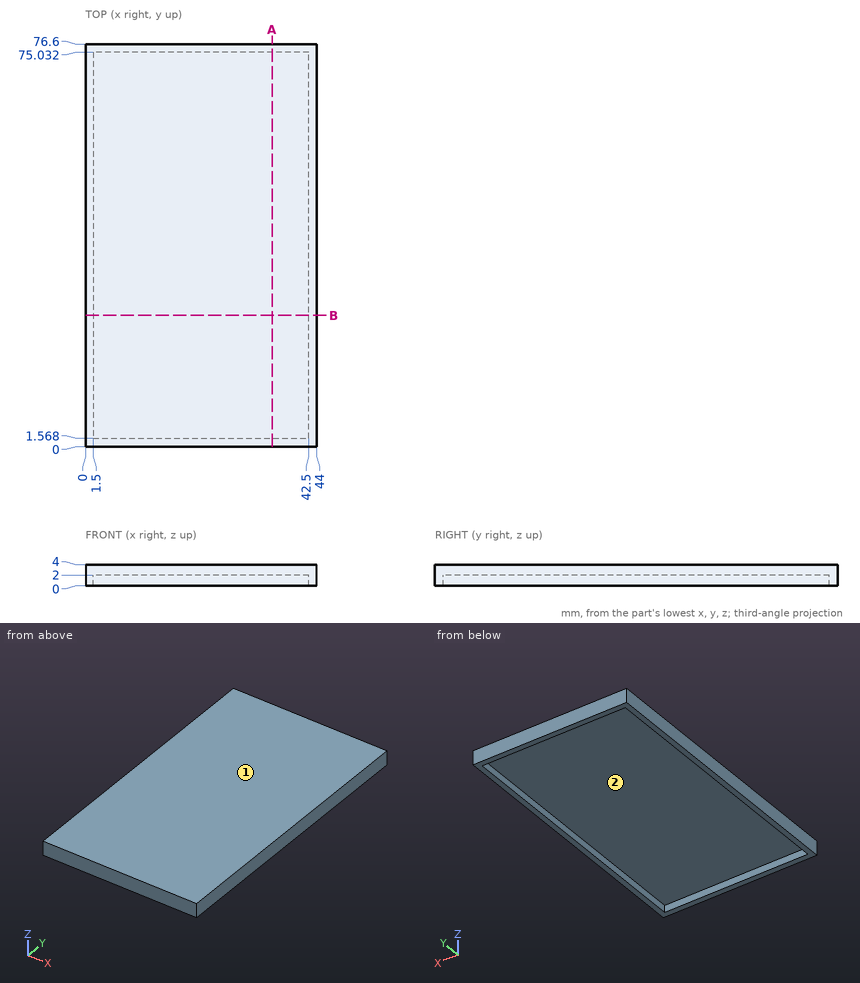
Can you work these out from the drawing? Everything is in mm from the part's minimum corner. Give positions to 0.01 mm unless a question says otherwise; leave off trailing zeros. Order: outer loops, then holes, each group sorted by start corner. A loop starts at its lowest first (then second) coordinate and runs counter-clockwise, first axis right, second up. Notation, with made-up numbers: M 44,24.5 L 102,24.5 A29 ccw 102,52.5 Z; hole C 34.5,-17 d10. An arc over 180 degrees is marked long. Write item = value, one per line. Start each with the question number.
Q1. We'd pull the mould along X, two halves only. Please class the marked faces 1 and 2: pulls with the +X half, pulls with the -X half, needs draft (parallel to the pull), parting line crosses it, or undercut.
Q2. Suppose I cut it at B-B (y = 25). Write out the boundary of the cut face in (x, z).
Q3. Will these pins go through, and if not, where does the flat tip stop? pin 1 Ø1.5 at (x, z) = (28.5, 2.5) entering from -Y; pin 2 Ø12.5 at (x, y) = (18, 26) entering from -Z.
Q4. I need wall thicknesses on probe 1 along Y at (x, z) = (40, 0.3); probe 2 along X at (y, z) = (32, 0.3); probe 3 along Z at (x, y) = (4.5, 34). Which ranges of each line are inside material? Lowest first, please. Write a range as [from, to].
Q5. Suppose I cut it at A-A (x = 35.5). Write out the boundary of the cut face in (y, z).
Check result:
q1.face_1 = needs draft
q1.face_2 = undercut
q2.outline = M 0,0 L 1.5,0 L 1.5,2 L 42.5,2 L 42.5,0 L 44,0 L 44,4 L 0,4 Z
q3.pin_1 = 0
q3.pin_2 = 2
q4.probe_1 = [0, 1.57], [75.03, 76.6]
q4.probe_2 = [0, 1.5], [42.5, 44]
q4.probe_3 = [2, 4]
q5.outline = M 0,0 L 1.57,0 L 1.57,2 L 75.03,2 L 75.03,0 L 76.6,0 L 76.6,4 L 0,4 Z
